Can you work these out from the drawing? Everything is in mm from the part's minimum corner. A direction names the side the tool comes from. Round coordinates to 2 decimals unless told otherwise and drop trailing zeros. Order: outer loops, then holes, each group sorted by start corner. A loop starts at its lowest first (then second) coordinate and runs counter-clockwise, first axis right, second up. Notation, with made-up numbers: (88.5, -33.5) - (108.5, -33.5) arc R16 cw to (108.5, -4.5) - close; hole circle Ø5 at (11.25, 51). An arc over 180 degrees is marked (long way). Answer as a JSON object with one key per item and string values.
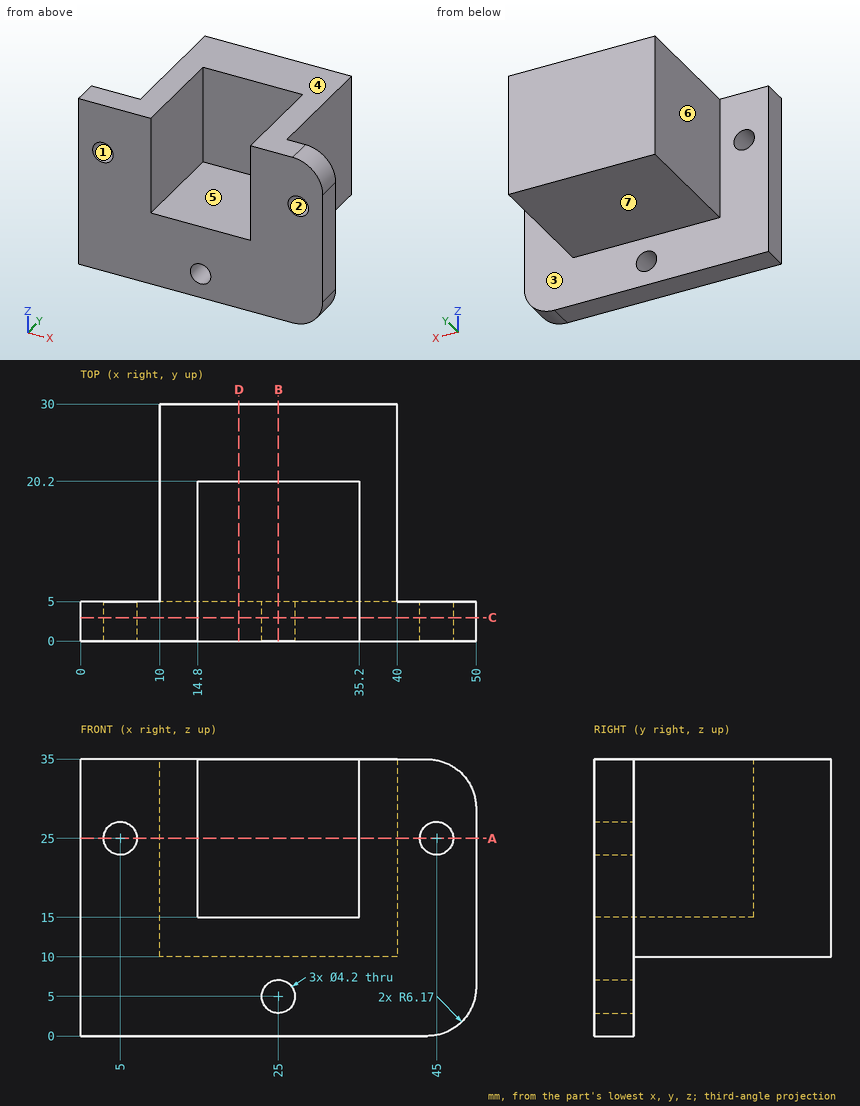
1. For the marked faces 5, 6 and 7, which set-ups out of +Z, -Z, +X, -X, +Y, -Y let a thin tool reach every point of the face, with its end or its side?
Responses:
{"face 5": "+Z, -Y", "face 6": "+Z, -Z, -X, +Y", "face 7": "-Z, +X, -X, +Y"}
2. Imagine slicing it at C-C (y = 3). List the corners of the cut face in (x, z) for me, plus the area to 3 significant figures.
Responses:
{"outline": "(0, 0) - (43.83, 0) arc R6.17 ccw to (50, 6.17) - (50, 28.83) arc R6.17 ccw to (43.83, 35) - (35.2, 35) - (35.2, 15) - (14.8, 15) - (14.8, 35) - (0, 35) - close; hole circle Ø4.2 at (5, 25); hole circle Ø4.2 at (25, 5); hole circle Ø4.2 at (45, 25)", "area": "1,280 mm2"}
3. Imagine slicing it at A-A (z = 25). List the corners of the cut face in (x, y) for me, plus the area to 3 significant figures.
Responses:
{"outline": "(0, 0) - (2.9, 0) - (2.9, 5) - (0, 5) - close; (7.1, 0) - (14.8, 0) - (14.8, 20.2) - (35.2, 20.2) - (35.2, 0) - (42.9, 0) - (42.9, 5) - (40, 5) - (40, 30) - (10, 30) - (10, 5) - (7.1, 5) - close; (47.1, 0) - (50, 0) - (50, 5) - (47.1, 5) - close", "area": "546 mm2"}
4. For P1, Ø5, axis at y = 14.5, z = 16.5, coming from the +X side; P2, Ø6, axis at x = 23.5, z = 28.5, coming from the -Y side; P3, Ø5, axis at x = 5, z = 25, coming from the +Y side, each with a flat end and sliding along its axis, tell me the tip position at first contact or that it passes through.
Responses:
{"P1": "x = 40", "P2": "y = 20.2", "P3": "y = 5"}
5. Thinking about a two-plate mould opening in Z: for the marked faces 1, 2, 3 and 4, which applies, pulls with the +Z half, pulls with the -Z half, needs draft (parallel to the pull), parting line crosses it, or undercut?
Responses:
{"face 1": "undercut", "face 2": "undercut", "face 3": "needs draft", "face 4": "pulls with the +Z half"}
6. Imagine slicing it at D-D (x = 20). List the corners of the cut face in (y, z) for me.
Responses:
{"outline": "(0, 0) - (5, 0) - (5, 10) - (30, 10) - (30, 35) - (20.2, 35) - (20.2, 15) - (0, 15) - close"}
7. If I drill on L1, parallel to X at y = 2.75, z = 25; L2, parallel to Z at x = 5, y = 2.7; L3, parallel to X at y = 10.5, z = 24, over which ranges is the centre line in solid material (lowest first)? Write a range as [from, to].
Responses:
{"L1": "[0, 2.9], [7.1, 14.8], [35.2, 42.9], [47.1, 50]", "L2": "[0, 22.9], [27.1, 35]", "L3": "[10, 14.8], [35.2, 40]"}
8. Imagine slicing it at B-B (x = 25). List the corners of the cut face in (y, z) for me.
Responses:
{"outline": "(0, 0) - (5, 0) - (5, 2.9) - (0, 2.9) - close; (0, 7.1) - (5, 7.1) - (5, 10) - (30, 10) - (30, 35) - (20.2, 35) - (20.2, 15) - (0, 15) - close"}
